Input: part model. Units: mm. Frame: model coordinates. Face numbers are marked on the shaded views. A direction names the side the tool comes from. Coordinates: 2 decimals unless noted, no trailing zeros. Answer as CSV lines item,"result".
from build123d import *

# Parameters (mm, degrees)
BOSS_EXTRUDE1_DEPTH              = 57.15
FILLET1_R                        = 3.175
F_1_2_0_5_DIAMETER_HOLE1_D       = 12.7
F_1_2_0_5_DIAMETER_HOLE1_DEPTH   = 45.72
F_1_2_0_5_DIAMETER_HOLE1_TIP     = 3.815464931
F_10_32_TAPPED_HOLE1_REACH       = 63.974
F_10_32_TAPPED_HOLE1_BORE_R      = 2.0193
F_29_0_136_DIAMETER_HOLE1_REACH  = 63.974
F_29_0_136_DIAMETER_HOLE1_BORE_R = 1.7272
CUT_EXTRUDE1_DEPTH               = 59.973007694
CIRPATTERN1_COUNT                = 6
SKETCH16_W                       = 25.4
SKETCH16_H                       = 25.4
CUT_EXTRUDE2_DEPTH               = 1.5875


with BuildPart() as part:
    # Sketch1 → Boss-Extrude1 (new body)
    with BuildSketch(Plane(origin=(0, 0, 0), x_dir=(1, 0, 0), z_dir=(0, 1, 0))):
        Polygon((10.998522628, 0), (5.499261314, 9.525), (-5.499261314, 9.525), (-10.998522628, 0), (-5.499261314, -9.525), (5.499261314, -9.525), align=None)
    extrude(amount=BOSS_EXTRUDE1_DEPTH)

    # Fillet1
    fillet1_edges = [part.edges().sort_by_distance(p)[0] for p in [
        (0, 0, 9.525),
        (-8.248891971, 0, 4.7625),
        (-8.248891971, 0, -4.7625),
        (0, 0, -9.525),
        (8.248891971, 0, -4.7625),
        (8.248891971, 0, 4.7625),
    ]]
    fillet(fillet1_edges, radius=FILLET1_R)

    # 1/2 (0.5) Diameter Hole1
    with Locations(Plane(origin=(0, 0, 0), x_dir=(-1, 0, 0), z_dir=(0, -1, 0))):
        with Locations((0, 0)):
            Hole(F_1_2_0_5_DIAMETER_HOLE1_D / 2, depth=F_1_2_0_5_DIAMETER_HOLE1_DEPTH)
            with Locations((0, 0, -(F_1_2_0_5_DIAMETER_HOLE1_DEPTH + F_1_2_0_5_DIAMETER_HOLE1_TIP / 2))):  # 118° drill point
                Cone(0, F_1_2_0_5_DIAMETER_HOLE1_D / 2, F_1_2_0_5_DIAMETER_HOLE1_TIP, mode=Mode.SUBTRACT)

    # #10-32 Tapped Hole1 bore → #10-32 Tapped Hole1 (cut, up to next)
    with BuildSketch(Plane(origin=(8.248891971, 0, 4.7625), x_dir=(0.49999999999999845, 0, -0.8660254037844396), z_dir=(0.8660254037844395, 0, 0.4999999999999984)), mode=Mode.PRIVATE) as f_10_32_tapped_hole1_sk1:
        with Locations((0, 22.225)):
            Circle(F_10_32_TAPPED_HOLE1_BORE_R)
    f_10_32_tapped_hole1_tool1 = extrude(f_10_32_tapped_hole1_sk1.sketch, amount=-F_10_32_TAPPED_HOLE1_REACH, mode=Mode.PRIVATE) & part.part
    add(f_10_32_tapped_hole1_tool1.solids().sort_by_distance((8.248892, 22.225, 4.7625))[0], mode=Mode.SUBTRACT)

    # #29 (0.136) Diameter Hole1 bore → #29 (0.136) Diameter Hole1 (cut, up to next)
    with BuildSketch(Plane(origin=(8.248891971, 0, 4.7625), x_dir=(0.49999999999999845, 0, -0.8660254037844396), z_dir=(0.8660254037844395, 0, 0.4999999999999984)), mode=Mode.PRIVATE) as f_29_0_136_diameter_hole1_sk1:
        with Locations((0, 38.4175)):
            Circle(F_29_0_136_DIAMETER_HOLE1_BORE_R)
    f_29_0_136_diameter_hole1_tool1 = extrude(f_29_0_136_diameter_hole1_sk1.sketch, amount=-F_29_0_136_DIAMETER_HOLE1_REACH, mode=Mode.PRIVATE) & part.part
    add(f_29_0_136_diameter_hole1_tool1.solids().sort_by_distance((8.248892, 38.4175, 4.7625))[0], mode=Mode.SUBTRACT)

    # Sketch13 → Cut-Extrude1 (cut, through all)
    with BuildSketch(Plane(origin=(0, 57.15, 0), x_dir=(1, 0, 0), z_dir=(0, 1, 0))):
        Polygon((-9.06849146, 11.262087957), (-5.89349146, 5.762826643), (-2.04400854, 7.985326643), (-5.21900854, 13.484587957), align=None)
    cut_extrude1 = extrude(amount=-CUT_EXTRUDE1_DEPTH, mode=Mode.SUBTRACT)

    # CirPattern1: Cut-Extrude1 ×6 about axis, 2 skipped
    cirpattern1_axis = Axis((0, 0, 0), (0, -1, 0))
    add([cut_extrude1.rotate(cirpattern1_axis, i * 360 / CIRPATTERN1_COUNT) for i in range(1, CIRPATTERN1_COUNT) if i not in (2, 3)], mode=Mode.SUBTRACT)

    # Sketch15 → Cut-Revolve4 (revolve, cut)
    with BuildSketch(Plane.XY, mode=Mode.PRIVATE) as cut_revolve4_sk:
        with BuildLine():
            Line((-10.998522628, 47.244), (-21.751479805, 47.244))
            Line((-21.751479805, 47.244), (-21.751479805, 61.468889452))
            Line((-21.751479805, 61.468889452), (0, 61.468889452))
            Line((0, 61.468889452), (0, 57.08956907))
            ThreePointArc((0, 57.08956907), (-7.699575937, 54.624764363), (-10.998522628, 47.244))
        make_face()
    revolve(cut_revolve4_sk.sketch.rotate(Axis((0, 61.468889452, 0), (0, -1, 0)), 90), axis=Axis((0, 61.468889452, 0), (0, -1, 0)), mode=Mode.SUBTRACT)

    # Sketch12 → Cut-Revolve6 (revolve, cut)
    with BuildSketch(Plane.XY, mode=Mode.PRIVATE) as cut_revolve6_sk:
        Polygon((7.9375, 35.316717762), (10.998522628, 37.084), (10.998522628, 24.0665), (7.9375, 25.833782238), align=None)
    revolve(cut_revolve6_sk.sketch.rotate(Axis((0, 0, 0), (0, 1, 0)), 90), axis=Axis((0, 0, 0), (0, 1, 0)), mode=Mode.SUBTRACT)

    # Sketch16 → Cut-Extrude2 (cut)
    with BuildSketch(Plane(origin=(8.248891971, 0, 4.7625), x_dir=(0.49999999999999845, 0, -0.8660254037844396), z_dir=(0.8660254037844395, 0, 0.4999999999999984))):
        with Locations((0, 54.2925)):
            Rectangle(SKETCH16_W, SKETCH16_H)
        with Locations((0, 6.35)):
            Rectangle(SKETCH16_W, SKETCH16_H)
    extrude(amount=-CUT_EXTRUDE2_DEPTH, mode=Mode.SUBTRACT)


solid = part.part
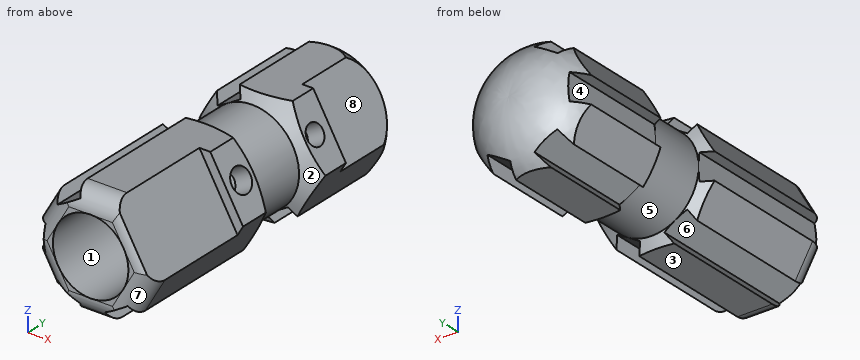
1. Reachability of the marked faces 1, 2, 3 and 4 from +Z, -Z, +X, -X, +Y, -Y: full face, straight path, thin tool, end or side. Return the list, or none.
Findings:
face 1,"-Y"
face 2,"none"
face 3,"-Z, +X, -X, +Y, -Y"
face 4,"-X, +Y, -Y"
2. Cut plane B-B (z = 4.5). State how many separate pieces and enclosed holes the cut face has, plus the area to 3 significant figures.
Findings:
separate pieces,"3"
enclosed holes,"0"
area,"390 mm2"
3. Ray query, line 1 along Z through (x, y) = (0, 22) (3 decimals); line 2 along Y through (x, z) = (1.5, -8); line 3 along X through (y, z) = (34, -0.75). Return the intervals inside material, ascending.
Findings:
line 1,"z = -9.525 to -6.35, 6.35 to 9.525"
line 2,"y = 0.46 to 25.72, 35.43 to 54.21"
line 3,"x = -7.9 to -6.31, 6.31 to 7.9"
4. Contact query for flat-ended pins moving along their axis: pin 1 (4 mm diameter, centred on x = -7.5, y = 42, fed in from +Z); pin 2 (2 mm diameter, centred on x = -9, y = 12, fed in from +Z); pin 3 (1.4 mm diameter, centred on x = -8.5, y = 11.5, fed in from -Z). Output: stop coordinate, or through.
Findings:
pin 1,"stops at z = 7.3"
pin 2,"stops at z = 5.19"
pin 3,"stops at z = -5.54"
5. Mould query, pull axis Z, two halves, no side actions, for the marked faces 5, 6, 7 and 8. Classes: released by +Z, released by -Z, zero draft, split by the parting line, or undercut.
Findings:
face 5,"split by the parting line"
face 6,"undercut"
face 7,"released by -Z"
face 8,"released by +Z"
